Verification items for the finished model (mm, model axes). Face numbers are marked on the shaded views. A direction names the side the tool comes from. Round coordinates to 2 decimals unless told otherwise and drop trailing zeros. Order: outer loops, then holes, each group sorted by start corner. A loop starts at its lowest first (then second) coordinate and runs counter-clockwise, first axis right, second up. Notation, with made-up numbers: (80, 66.5) -> (108, 66.5) arc R11 cw to (108, 87.5) -> close; hole circle Ø10 at (86.25, 56). An arc over 180 degrees is marked (long way). Put each result on its own line as item: value.
from build123d import *

# Parameters (mm, degrees)
EXTRUDE_1_DEPTH      = 25
EXTRUDE_1_DEPTH_BACK = 1
SKETCH_1_R           = 4
EXTRUDE_2_DEPTH      = 7
EXTRUDE_2_DEPTH_BACK = 1
SKETCH_2_R           = 2.5
EXTRUDE_3_DEPTH      = 2
EXTRUDE_START        = 2
SKETCH_2_3_R         = 6
SKETCH_2_3_R_2       = 2.5
EXTRUDE_4_DEPTH      = 2
SKETCH_4_W           = 0.8
SKETCH_4_H           = 0.6
SKETCH_5_R           = 8.5
EXTRUDE_5_DEPTH      = 20.2
SKETCH_6_W           = 1
SKETCH_6_H           = 0.65
FILLET_2_R           = 2


with BuildPart() as part:
    # 草图1 → 凸台-拉伸1 (new, two sides: drawn at the far end of the back side and taken through both)
    with BuildSketch(Plane.XY.offset(-EXTRUDE_1_DEPTH_BACK)):
        Circle(SKETCH_1_R)
        with BuildLine():
            Line((-2, -1.5), (-2, 1.5))
            ThreePointArc((-2, 1.5), (2.5, 0), (-2, -1.5))
        make_face(mode=Mode.SUBTRACT)
    extrude(amount=EXTRUDE_1_DEPTH + EXTRUDE_1_DEPTH_BACK)

    # 草图1<3> → 凸台-拉伸2 (add, two sides: drawn at the far end of the back side and taken through both)
    with BuildSketch(Plane.XY.offset(-EXTRUDE_2_DEPTH_BACK)):
        with BuildLine():
            Line((-1.5, 5.4), (-1.5, 3.708099244))
            ThreePointArc((-1.5, 3.708099244), (0, 4), (1.5, 3.708099244))
            Line((1.5, 3.708099244), (1.5, 5.4))
            Line((1.5, 5.4), (-1.5, 5.4))
        make_face()
        with BuildLine():
            Line((5.4, 1.5), (3.708099244, 1.5))
            ThreePointArc((3.708099244, 1.5), (4, 0), (3.708099244, -1.5))
            Line((3.708099244, -1.5), (5.4, -1.5))
            Line((5.4, -1.5), (5.4, 1.5))
        make_face()
    extrude(amount=EXTRUDE_2_DEPTH + EXTRUDE_2_DEPTH_BACK)

    # 草图2 → 凸台-拉伸3 (add)
    with BuildSketch(Plane(origin=(0, 0, -1), x_dir=(-1, 0, 0), z_dir=(0, 0, -1))):
        Circle(SKETCH_2_R)
    extrude(amount=-EXTRUDE_3_DEPTH)

    # 草图2<3> → 凸台-拉伸4 (add)
    # profile 1 of 2: a face of its own
    with BuildSketch(Plane(origin=(0, 0, -1), x_dir=(-1, 0, 0), z_dir=(0, 0, -1)).offset(EXTRUDE_START)):
        Circle(SKETCH_2_3_R)
        Circle(SKETCH_2_3_R_2, mode=Mode.SUBTRACT)
    # profile 2 of 2: a face of its own
    with BuildSketch(Plane(origin=(0, 0, -1), x_dir=(-1, 0, 0), z_dir=(0, 0, -1)).offset(EXTRUDE_START)):
        Circle(SKETCH_2_3_R_2)
    extrude(amount=-EXTRUDE_4_DEPTH)

    # 草图4 → 切除-旋转3 (revolve, cut)
    with BuildSketch(Plane(origin=(0, 0, 0), x_dir=(0, 0, -1), z_dir=(1, 0, 0)), mode=Mode.PRIVATE) as cut_revolve_3_sk:
        with Locations((-7.4, 3.7)):
            Rectangle(SKETCH_4_W, SKETCH_4_H)
    revolve(cut_revolve_3_sk.sketch.rotate(Axis((0, 0, 0), (0, 0, 1)), 90), axis=Axis((0, 0, 0), (0, 0, 1)), mode=Mode.SUBTRACT)

    # 草图5 → 凸台-拉伸5 (add)
    with BuildSketch(Plane(origin=(0, 0, -3), x_dir=(-1, 0, 0), z_dir=(0, 0, -1))):
        Circle(SKETCH_5_R)
    extrude(amount=EXTRUDE_5_DEPTH)

    # 草图6 → 切除-旋转4 (revolve, cut)
    with BuildSketch(Plane(origin=(0, 0, 0), x_dir=(0, 0, -1), z_dir=(1, 0, 0)), mode=Mode.PRIVATE) as cut_revolve_4_sk:
        with Locations((20.7, 8.175)):
            Rectangle(SKETCH_6_W, SKETCH_6_H)
    revolve(cut_revolve_4_sk.sketch.rotate(Axis((0, 0, 0), (0, 0, -1)), 90), axis=Axis((0, 0, 0), (0, 0, -1)), mode=Mode.SUBTRACT)

    # 圆角2
    fillet_2_edges = [part.edges().sort_by_distance(p)[0] for p in [
        (6, 0, -3),
    ]]
    fillet(fillet_2_edges, radius=FILLET_2_R - 0.0001)  # a hair under: the kernel refuses the full size


solid = part.part
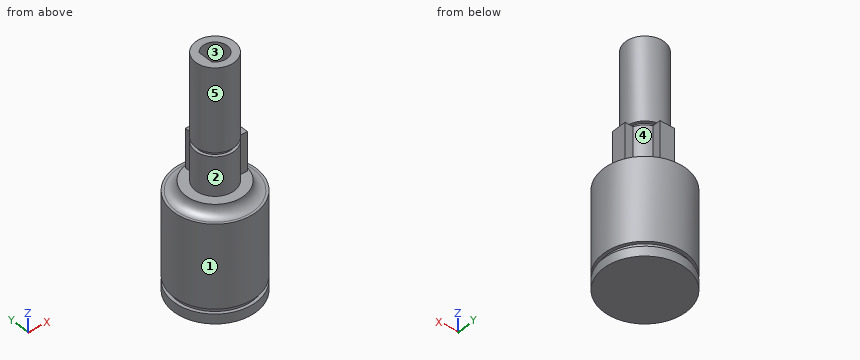
Item 1: Tool access check on the marked faces 1 and 2. Record the directions out of +Z, -Z, +X, -X, +Y, -Y that give a thin tool (end or side, any length) a straight path to the whole face; none if there is none.
Check sheet entries:
face 1: +Z, -Z
face 2: +Z
Item 2: Release check for a two-part mould opening along X. For the marked faces 3, 4 and 5 record: +X half, -X half, draft (parallel to the pull), parting line (faces both ways), or undercut.
Check sheet entries:
face 3: undercut
face 4: +X half
face 5: parting line
Item 3: Section check D-D on z = -1.5. Record the boundary of the cut face in (x, y), then the cut area to 3 significant figures.
Check sheet entries:
outline: circle Ø12.13 at (0, 0)
area: 116 mm^2
Item 4: Gauge pin test, flat ends, axial feed: pin 1 Ø1.5 at (x, y) = (4.5, -2) entering from +Z; pin 2 Ø1.5 at (y, z) = (-5, -15.5) entering from -X; pin 3 Ø0.8 at (y, z) = (5, 5) entering from +X. Record the tip position at first contact, or that the pin passes through.
Check sheet entries:
pin 1: stops at z = 7
pin 2: stops at x = -7.36
pin 3: stops at x = 1.5
Item 5: Section check C-C on z = 14. Record the boundary of the cut face in (x, y).
Check sheet entries:
outline: circle Ø8 at (0, 0); hole (-2, -1.5) arc R2.5 ccw (long way) to (-2, 1.5) -> close
Item 6: Material ranges on L1, parallel to X at y = 0, z = 12; L2, parallel to Y at x = 0, z = 14.5; L3, parallel to Y at x = 7.5, z = -3.5, recorded low to high. Write a range as [from, to].
Check sheet entries:
L1: x = [-4, -2], [2.5, 4]
L2: y = [-4, -2.5], [2.5, 4]
L3: y = [-4, 4]
